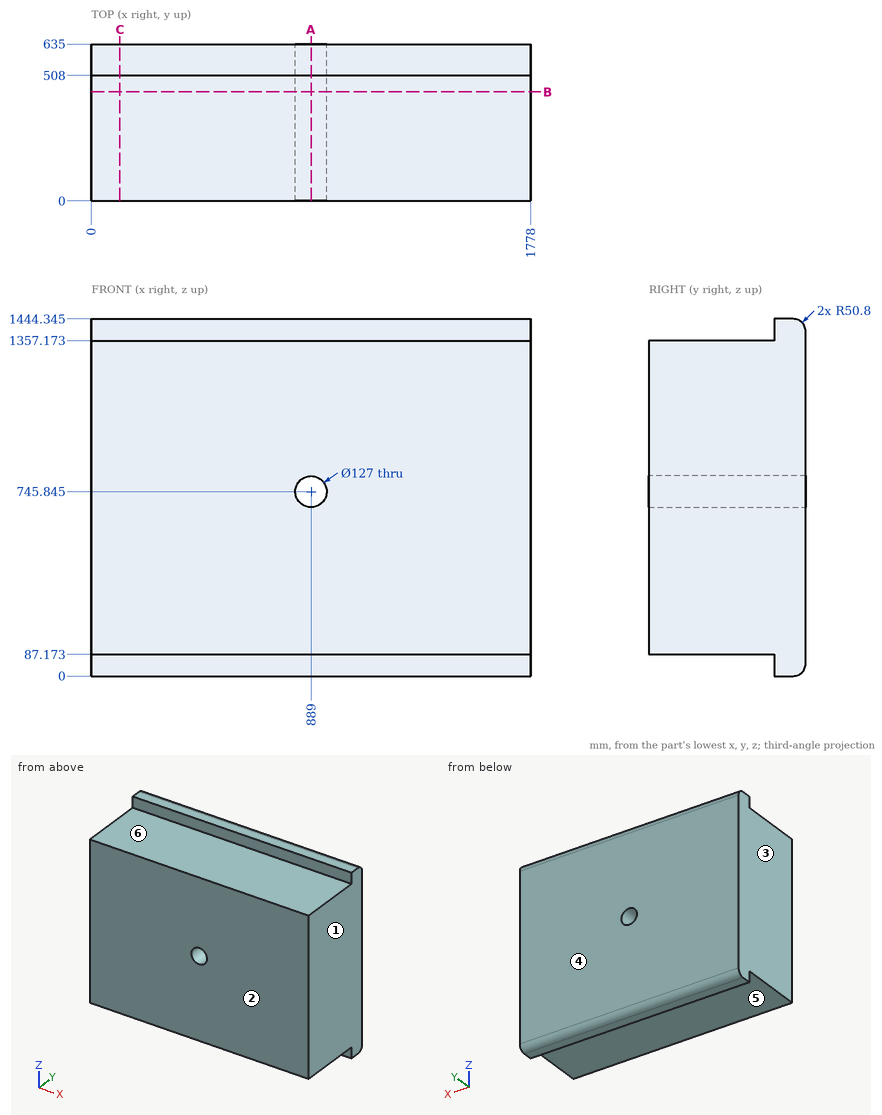
Check sheet for the drawn part. Datum: minimum x, y, z corner. Units: mm. A direction names the side the tool comes from. Give positions to 0.01 mm unless a question says otherwise; leave off trailing zeros. Order: outer loops, then holes, each group sorted by start corner. A loop starts at its lowest first (then second) coordinate and runs counter-clockwise, first axis right, second up. Notation, with made-up numbers: (-26.5, 56.5) - (21.5, 56.5) arc R27 cw to (21.5, 87.5) - close; hole circle Ø4 at (3, -14). An arc over 180 degrees is marked (long way). Answer in a Markdown table with one row per item. Add a question column.
Q1. Tool access check on the marked faces 4, 5 and 6. Record the directions out of +Z, -Z, +X, -X, +Y, -Y that give a thin tool (end or side, any length) a straight path to the whole face; none if there is none.
Q2. Mould release check, pull along X, two halves, no side actions. Record for the marked faces 1, 2 and 3: pulls with the +X half, pulls with the -X half, needs draft (parallel to the pull), parting line crosses it, or undercut.
Q3. Cross-section at B-B, the plane y = 441. Enter the section's corners in (x, z) (1 decimal), then the cut area to 3 significant figures.
Q4. Cross-section at C-C, the plane x = 116. Enter the section's corners in (y, z) (1 decimal), then the cut area to 3 significant figures.
Q5. Cross-section at A-A, the plane x = 889. Enter the section's corners in (y, z) (1 decimal).
Q6. Gauge pin test, flat ends, axial feed: pin 1 (3 mm diameter, centred on y = 554, z = 667, fed in from -X); pin 2 (3 mm diameter, centred on x = 1146.5, y = 288, fed in from +Z). Record the tip position at first contact, or that the pin passes through.
Q7. Material ranges on probe 1 along Z at (x, y) = (1142, 304); probe 2 along Z at (x, y) = (918, 499) (1 decimal); probe 3 along X at (y, z) = (331.5, 804), recorded low to high. Write a range as from..to.
Check values:
| question | item | result |
|---|---|---|
| 1 | face 4 | +Z, -Z, +X, -X, +Y |
| 1 | face 5 | -Z, +X, -X, -Y |
| 1 | face 6 | +Z, +X, -X, -Y |
| 2 | face 1 | pulls with the +X half |
| 2 | face 2 | needs draft |
| 2 | face 3 | pulls with the -X half |
| 3 | outline | (0, 87.2) - (1778, 87.2) - (1778, 1357.2) - (0, 1357.2) - close; hole circle Ø127 at (889, 745.8) |
| 3 | area | 2,250,000 mm^2 |
| 4 | outline | (0, 87.2) - (508, 87.2) - (508, 0) - (584.2, 0) arc R50.8 ccw to (635, 50.8) - (635, 1393.5) arc R50.8 ccw to (584.2, 1444.3) - (508, 1444.3) - (508, 1357.2) - (0, 1357.2) - close |
| 4 | area | 827,000 mm^2 |
| 5 | outline | (0, 87.2) - (508, 87.2) - (508, 0) - (584.2, 0) arc R50.8 ccw to (635, 50.8) - (635, 682.3) - (0, 682.3) - close; (0, 809.3) - (635, 809.3) - (635, 1393.5) arc R50.8 ccw to (584.2, 1444.3) - (508, 1444.3) - (508, 1357.2) - (0, 1357.2) - close |
| 6 | pin 1 | stops at x = 0 |
| 6 | pin 2 | stops at z = 1357.17 |
| 7 | probe 1 | z = 87.17..1357.17 |
| 7 | probe 2 | z = 87.2..689.4, 802.3..1357.2 |
| 7 | probe 3 | x = 0..863.5, 914.5..1778 |
